Build history of the part. All positions in model axes, mm. A direction names the side the tool comes from. Give positions to 0.01 mm unless a question says otherwise; leave off trailing zeros. Write each loop counter-clockwise with the first axis right and the second up, starting at its lowest first coordinate (ties: lowest second). Pieces come first, ordered by that corner, then holes. Notation, with made-up numbers: (49, 20.5) -> (77, 20.5) arc R13 cw to (77, 24.5) -> close; hole circle Ø9 at (67, 47.25). An arc over 180 degrees is marked (long way). Put each result on its own line as item: value. Start each with the question number.
Item 1: Two-plate mould, pull along X, no slides. Class faces 4 (the flat face through (14.05, 2, 0)), 5 (the flat face through (15.5, 5.3, -0.3)), 6 (the flat face through (-10, 4.8, -5)): pulls with the +X half, pulls with the -X half, needs draft (parallel to the pull), parting line crosses it, or undercut.
Item 2: Slice it at C-C, the plane y = 2.25. List the corners of the cut face in (x, z), plus the area to 3 significant figures.
Item 3: Slice it at A-A, the plane y = 4.25. List the corners of the cut face in (x, z).
Item 4: Tool access for faces 1 (the flat face through (15.4, 5.3, -2.24)), 2 (the cylindrical face through (12.83, 5.36, 2.54)), 3 (the flat face through (15.5, 5.3, -2.84)): list every direction of +Z, -Z, +X, -X, +Y, -Y with a clear straight run to the whole face (end or side of a thin tool).
Item 5: Flat gauge pins, fed straight in: pin 1 Ø2 at (x, z) = (2, 0) entering from -Y; pin 2 Ø0.6 at (x, z) = (-2, 6) entering from +Y; pin 3 Ø1.8 at (x, y) = (12.5, 3) entering from +Z; pin 4 Ø0.6 at (y, z) = (6.5, -2.5) entering from +X. Where does each tip first touch, or does it go through?
Item 6: Slice it at B-B, the plane x = -4.5. List the corners of the cut face in (y, z), plus the area to 3 significant figures.
Item 7: Drill centre lines: line 1 along X through (y, z) = (7.25, -5.25); line 2 along X through (y, z) = (2, 1); line 3 along X through (y, z) = (0.85, 0). Where is each one in solid material? Low to high.
```python
from build123d import *

# Parameters (mm, degrees)
SKETCH_1_W             = 31.1
SKETCH_1_H             = 14.1
EXTRUDE_1_DEPTH        = 1
SKETCH_2_W             = 16
SKETCH_2_H             = 12.7
EXTRUDE_2_DEPTH        = 6.3
SKETCH_3_R             = 1.75
CUT_EXTRUDE_1_DEPTH    = 19.198763694
SKETCH_4_R             = 1.4
EXTRUDE_3_DEPTH        = 5.7
FILLET_1_R             = 1.2
SKETCH_5_W             = 2.3
SKETCH_5_H             = 7
EXTRUDE_4_DEPTH        = 2.8
SKETCH_6_W             = 0.6
SKETCH_6_H             = 0.6
PATTERN_LINEAR_1_COUNT = 2
PATTERN_LINEAR_1_PITCH = 2.54
PATTERN_LINEAR_2_COUNT = 2
PATTERN_LINEAR_2_PITCH = 2.54
CHAMFER_1_SIZE         = 0.25
SKETCH_7_W             = 2.808166855
SKETCH_7_H             = 1.049205199
SKETCH_7_W_2           = 2.530436068
EXTRUDE_5_DEPTH        = 0.5
SKETCH_8_R             = 0.15
PATTERN_LINEAR_3_COUNT = 4
PATTERN_LINEAR_3_PITCH = 3.3
SKETCH_9_W             = 1.2
SKETCH_9_H             = 1.2
SKETCH_9_H_2           = 1.828804168
CUT_EXTRUDE_2_DEPTH    = 2.5


with BuildPart() as part:
    # Эскиз1 → Бобышка-Вытянуть1 (new body)
    with BuildSketch(Plane(origin=(0, 0, 0), x_dir=(1, 0, 0), z_dir=(0, 1, 0))):
        Rectangle(SKETCH_1_W, SKETCH_1_H)
    extrude(amount=EXTRUDE_1_DEPTH)

    # Эскиз2 → Бобышка-Вытянуть2 (add)
    with BuildSketch(Plane(origin=(0, 1, 0), x_dir=(1, 0, 0), z_dir=(0, 1, 0))):
        with Locations((-4.55, 0)):
            Rectangle(SKETCH_2_W, SKETCH_2_H)
    extrude(amount=EXTRUDE_2_DEPTH)

    # Эскиз3 → Вырез-Вытянуть1 (cut, through all)
    with BuildSketch(Plane(origin=(0, 1, 0), x_dir=(1, 0, 0), z_dir=(0, 1, 0))):
        with Locations(Location((7.2, 0, 0), (0, 0, 270))):
            Circle(SKETCH_3_R)
    extrude(amount=-CUT_EXTRUDE_1_DEPTH, mode=Mode.SUBTRACT)

    # Эскиз4 → Бобышка-Вытянуть3 (add)
    with BuildSketch(Plane(origin=(0, 1, 0), x_dir=(1, 0, 0), z_dir=(0, 1, 0))):
        with Locations(Location((7.15, -4.25, 0), (0, 0, 270))):
            Circle(SKETCH_4_R)
    extrude(amount=EXTRUDE_3_DEPTH)

    # Скругление1
    fillet_1_edges = [part.edges().sort_by_distance(p)[0] for p in [
        (7.15, 6.7, 2.85),
    ]]
    fillet(fillet_1_edges, radius=FILLET_1_R)

    # Эскиз5 → Бобышка-Вытянуть4 (add)
    with BuildSketch(Plane(origin=(0, 1, 0), x_dir=(1, 0, 0), z_dir=(0, 1, 0))):
        with Locations((12.9, 0)):
            Rectangle(SKETCH_5_W, SKETCH_5_H)
    extrude(amount=EXTRUDE_4_DEPTH)

    # По траектории1: sweep along a curve in space
    with BuildLine() as sweep_1_path:
        Line((12.9, 3.8, 0), (12.9, 4.8, 0))
        ThreePointArc((12.9, 4.8, 0), (13.046446609, 5.153553391, 0), (13.4, 5.3, 0))
        Line((13.4, 5.3, 0), (20.15, 5.3, 0))
    # Эскиз6 → По траектории1 (sweep)
    with BuildSketch(Plane(origin=(0, 3.8, 0), x_dir=(1, 0, 0), z_dir=(0, 1, 0))):
        with Locations((12.9, 0)):
            Rectangle(SKETCH_6_W, SKETCH_6_H)
    sweep_1 = sweep(path=sweep_1_path.line)

    # Линейный массив1: По траектории1 ×2
    with Locations(*[(0, 0, i * PATTERN_LINEAR_1_PITCH) for i in range(1, PATTERN_LINEAR_1_COUNT)]):
        add(sweep_1)

    # Линейный массив2: По траектории1 ×2
    with Locations(*[(0, 0, -i * PATTERN_LINEAR_2_PITCH) for i in range(1, PATTERN_LINEAR_2_COUNT)]):
        add(sweep_1)

    # Фаска1
    chamfer_1_edges = [part.edges().sort_by_distance(p)[0] for p in [
        (20.15, 5.3, -2.24),
        (20.15, 5, 0),
        (20.15, 5.3, -0.3),
        (20.15, 5.6, 0),
        (20.15, 5.3, 0.3),
        (20.15, 5, 2.54),
        (20.15, 5.3, 2.24),
        (20.15, 5.6, 2.54),
        (20.15, 5.3, 2.84),
        (20.15, 5, -2.54),
        (20.15, 5.3, -2.84),
        (20.15, 5.6, -2.54),
    ]]
    chamfer(chamfer_1_edges, length=CHAMFER_1_SIZE)

    # Эскиз7 → Бобышка-Вытянуть5 (add)
    with BuildSketch(Plane(origin=(0, 1, 0), x_dir=(1, 0, 0), z_dir=(0, 1, 0))):
        with Locations((6.287343289, 5.170597973)):
            Rectangle(SKETCH_7_W, SKETCH_7_H)
        with Locations((9.944131996, 5.170597973)):
            Rectangle(SKETCH_7_W_2, SKETCH_7_H)
    extrude(amount=EXTRUDE_5_DEPTH)

    # По траектории2: sweep along a curve in space
    with BuildLine() as sweep_2_path:
        Line((-12.55, 3.6, -5), (-12.999732268, 3.6, -5))
        ThreePointArc((-12.999732268, 3.6, -5), (-13.353285658, 3.453553391, -5), (-13.499732268, 3.1, -5))
        Line((-13.499732268, 3.1, -5), (-13.499732268, 1, -5))
    # Эскиз8 → По траектории2 (sweep)
    with BuildSketch(Plane.ZY.offset(12.55)):
        with Locations((-5, 3.6)):
            Circle(SKETCH_8_R)
    sweep_2 = sweep(path=sweep_2_path.line)

    # Линейный массив3: По траектории2 ×4
    with Locations(*[(0, 0, i * PATTERN_LINEAR_3_PITCH) for i in range(1, PATTERN_LINEAR_3_COUNT)]):
        add(sweep_2)

    # Эскиз9 → Вырез-Вытянуть2 (cut)
    with BuildSketch(Plane(origin=(0, 7.3, 0), x_dir=(1, 0, 0), z_dir=(0, 1, 0))):
        with Locations((3.45, 0)):
            Rectangle(SKETCH_9_W, SKETCH_9_H)
        with Locations((0.75, 0)):
            Rectangle(SKETCH_9_W, SKETCH_9_H)
        with Locations((-1.95, 0)):
            Rectangle(SKETCH_9_W, SKETCH_9_H)
        with Locations((-4.65, 0)):
            Rectangle(SKETCH_9_W, SKETCH_9_H)
        with Locations((-7.35, 0)):
            Rectangle(SKETCH_9_W, SKETCH_9_H)
        with Locations((-10.05, 0)):
            Rectangle(SKETCH_9_W, SKETCH_9_H)
        with Locations((3.45, 2.7)):
            Rectangle(SKETCH_9_W, SKETCH_9_H)
        with Locations((0.75, 2.7)):
            Rectangle(SKETCH_9_W, SKETCH_9_H)
        with Locations((-1.95, 2.7)):
            Rectangle(SKETCH_9_W, SKETCH_9_H)
        with Locations((-4.65, 2.7)):
            Rectangle(SKETCH_9_W, SKETCH_9_H)
        with Locations((-7.35, 2.7)):
            Rectangle(SKETCH_9_W, SKETCH_9_H)
        with Locations((-10.05, 2.7)):
            Rectangle(SKETCH_9_W, SKETCH_9_H)
        with Locations((3.45, -2.7)):
            Rectangle(SKETCH_9_W, SKETCH_9_H)
        with Locations((0.75, -2.7)):
            Rectangle(SKETCH_9_W, SKETCH_9_H)
        with Locations((-1.95, -2.7)):
            Rectangle(SKETCH_9_W, SKETCH_9_H)
        with Locations((-4.65, -2.7)):
            Rectangle(SKETCH_9_W, SKETCH_9_H)
        with Locations((-7.35, -2.7)):
            Rectangle(SKETCH_9_W, SKETCH_9_H)
        with Locations((-10.05, -2.7)):
            Rectangle(SKETCH_9_W, SKETCH_9_H)
        with Locations((-10.05, 5.435597916)):
            Rectangle(SKETCH_9_W, SKETCH_9_H_2)
        with Locations((-4.65, 5.435597916)):
            Rectangle(SKETCH_9_W, SKETCH_9_H_2)
        with Locations((-1.95, 5.435597916)):
            Rectangle(SKETCH_9_W, SKETCH_9_H_2)
        with Locations((-1.95, -5.435597916)):
            Rectangle(SKETCH_9_W, SKETCH_9_H_2)
        with Locations((-4.65, -5.435597916)):
            Rectangle(SKETCH_9_W, SKETCH_9_H_2)
        with Locations((-10.05, -5.435597916)):
            Rectangle(SKETCH_9_W, SKETCH_9_H_2)
    extrude(amount=-CUT_EXTRUDE_2_DEPTH, mode=Mode.SUBTRACT)


solid = part.part
```
Values follow:
1. face 4: pulls with the +X half
1. face 5: needs draft
1. face 6: undercut
2. outline: circle Ø0.3 at (-13.5, -5); circle Ø0.3 at (-13.5, -1.7); circle Ø0.3 at (-13.5, 1.6); circle Ø0.3 at (-13.5, 4.9); (-12.55, -6.35) -> (3.45, -6.35) -> (3.45, 6.35) -> (-12.55, 6.35) -> close; circle Ø2.8 at (7.15, 4.25); (11.75, -3.5) -> (14.05, -3.5) -> (14.05, 3.5) -> (11.75, 3.5) -> close
2. area: 226 mm2
3. outline: (-12.55, -6.35) -> (3.45, -6.35) -> (3.45, 6.35) -> (-12.55, 6.35) -> close; circle Ø2.8 at (7.15, 4.25); (12.6, -2.84) -> (13.2, -2.84) -> (13.2, -2.24) -> (12.6, -2.24) -> close; (12.6, -0.3) -> (13.2, -0.3) -> (13.2, 0.3) -> (12.6, 0.3) -> close; (12.6, 2.24) -> (13.2, 2.24) -> (13.2, 2.84) -> (12.6, 2.84) -> close
4. face 1: +X, +Y
4. face 2: +Z, -Z, +Y
4. face 3: -Z, +X, +Y
5. pin 1: y = 0
5. pin 2: y = 4.8
5. pin 3: z = 3.5
5. pin 4: x = 2.85
6. outline: (0, -7.05) -> (1, -7.05) -> (1, -6.35) -> (4.8, -6.35) -> (4.8, -4.52) -> (7.3, -4.52) -> (7.3, -3.3) -> (4.8, -3.3) -> (4.8, -2.1) -> (7.3, -2.1) -> (7.3, -0.6) -> (4.8, -0.6) -> (4.8, 0.6) -> (7.3, 0.6) -> (7.3, 2.1) -> (4.8, 2.1) -> (4.8, 3.3) -> (7.3, 3.3) -> (7.3, 4.52) -> (4.8, 4.52) -> (4.8, 6.35) -> (1, 6.35) -> (1, 7.05) -> (0, 7.05) -> close
6. area: 76.0 mm2
7. line 1: -12.55 to -10.65, -9.45 to -5.25, -4.05 to -2.55, -1.35 to 3.45
7. line 2: -12.55 to 3.45, 11.75 to 14.05
7. line 3: -15.55 to 5.45, 8.95 to 15.55
